```python
from build123d import *

# Parameters (mm, degrees)
F0_W     = 140
F0_H     = 60
F1_DEPTH = 60
F3_R     = 10.210921
F6_DEPTH = 10
F4_R     = 10
F7_DEPTH = 110.6
F5_R     = 10
F8_DEPTH = 10


with BuildPart() as f1:
    # F0 (on Top) → F1 (new body)
    with BuildSketch(Plane.XY):
        with Locations((2.316078, 0)):
            Rectangle(F0_W, F0_H)
    extrude(amount=F1_DEPTH)

    # F3 (on face) → F6 (join)
    with BuildSketch(Plane.XY.offset(60)):
        with BuildLine():
            ThreePointArc((-48.704213, 0), (-38.600937, -10.421296), (-28.284551, -0.210921))
            ThreePointArc((-28.284551, -0.210921), (-38.390005, 9.999455), (-48.704213, 0))
        make_face()
        with Locations((-38.495471, -0.210921)):
            Circle(F3_R)
    extrude(amount=F6_DEPTH)

    # F4 (on face) → F7 (cut)
    with BuildSketch(Plane.XY.offset(60)):
        Circle(F4_R)
    extrude(amount=-F7_DEPTH, mode=Mode.SUBTRACT)

    # F5 (on face) → F8 (cut)
    with BuildSketch(Plane.XY.offset(60)):
        with Locations((39.79122, -0.047711)):
            Circle(F5_R)
    extrude(amount=-F8_DEPTH, mode=Mode.SUBTRACT)


solid = f1.part
```
Model file for the job. Use its own axes, mm. A direction names the side the tool comes from. Give positions to 0.01 mm unless a question says otherwise; leave off trailing zeros. Write each loop counter-clockwise with the first axis right and the second up, starting at its lowest first coordinate (ties: lowest second). Pieces come first, ordered by that corner, then holes. Notation, with made-up numbers: (78, 78.25) -> (90, 78.25) arc R12 cw to (90, 83.25) -> close; hole circle Ø6 at (84, 34.25). An arc over 180 degrees is marked (long way). Use CSV: the item, a comma, the result in double quotes. Start each with the question number.
1) Tool access for faces 4 (the flat face through (1, 30, 30)), 5 (the flat face through (40, 0, 50)): list every direction of +Z, -Z, +X, -X, +Y, -Y with a clear straight run to the whole face (end or side of a thin tool).
2) Drill centre lines: L1, parallel to Y at x = 0, z = 47; L2, parallel to Z at x = -5.5, y = 17.5; L3, parallel to X at y = 1, z = 7.5. Where is each one in solid material? Low to high.
3) Cut at D-D on z = 56.5. List the corners of the cut face in (x, y).
4) Cut at B-B on z = 7.5. List the corners of the cut face in (x, y).
5) Two-plate mould, pull along X, no slides. Class faces 1 (the cylindrical face through (-2.17, -9.76, 30.42)), 2 (the cylindrical face through (-48.7, 0.2, 64.9)), 3 (the flat face through (1, 14, 0)): released by +X, released by -X, zero draft, split by the parting line, or undercut.
6) Cut at C-C on y = -6.5. List the corners of the cut face in (x, z).
7) Cut at A-A on x = 0. List the corners of the cut face in (y, z).
8) Pin check, flat tip, straight feed: P1, Ø1, axis at x = 43.5, y = 17.5, coming from the +Z side. Stop position of the tip, or through.
Final values:
1,face 4,"+Z, -Z, +X, -X, +Y"
1,face 5,"+Z"
2,L1,"y = -30 to -10, 10 to 30"
2,L2,"z = 0 to 60"
2,L3,"x = -67.68 to -9.95, 9.95 to 72.32"
3,outline,"(-67.68, -30) -> (72.32, -30) -> (72.32, 30) -> (-67.68, 30) -> close; hole circle Ø20 at (0, 0); hole circle Ø20 at (39.79, -0.05)"
4,outline,"(-67.68, -30) -> (72.32, -30) -> (72.32, 30) -> (-67.68, 30) -> close; hole circle Ø20 at (0, 0)"
5,face 1,"undercut"
5,face 2,"split by the parting line"
5,face 3,"zero draft"
6,outline,"(-67.68, 0) -> (-7.6, 0) -> (-7.6, 60) -> (-30.45, 60) -> (-30.45, 70) -> (-46.54, 70) -> (-46.54, 60) -> (-67.68, 60) -> close; (7.6, 0) -> (72.32, 0) -> (72.32, 60) -> (47.43, 60) -> (47.43, 50) -> (32.15, 50) -> (32.15, 60) -> (7.6, 60) -> close"
7,outline,"(-30, 0) -> (-10, 0) -> (-10, 60) -> (-30, 60) -> close; (10, 0) -> (30, 0) -> (30, 60) -> (10, 60) -> close"
8,P1,"stops at z = 60"
